Build history of the part. All positions in model axes, mm. Give positions to 0.01 mm unless a question says otherwise; leave off trailing zeros. Order: outer loops, then holes, each group sorted by start corner. A loop starts at its lowest first (then second) coordinate and runs counter-clockwise, first axis right, second up. Notation, with made-up numbers: (-34, 51.5) - (-26, 51.5) arc R25 ccw to (-26, 66.5) - close; hole circle Ø7 at (60, -30.75). An arc over 180 degrees is marked (long way). Answer in a Markdown table with one row per item.
```python
from build123d import *

# Parameters (mm, degrees)
BOSS_EXTRU_1_DEPTH      = 8
ENL_V_MAT_EXTRU_1_DEPTH = 4
CONG_2_R                = 10


with BuildPart() as part:
    # Esquisse1 → Boss.-Extru.1 (new body)
    with BuildSketch(Plane.XY):
        with BuildLine():
            Line((3.721082869, 15), (1.264283788, 21.75))
            Line((1.264283788, 21.75), (-1.264283788, 21.75))
            Line((-1.264283788, 21.75), (-3.721082869, 15))
            Line((-3.721082869, 15), (-53.721082869, 15))
            Line((-53.721082869, 15), (-53.721082869, -15))
            Line((-53.721082869, -15), (27.823144925, -15))
            Line((27.823144925, -15), (33.823144925, -19.5))
            ThreePointArc((33.823144925, -19.5), (35.323144925, -20), (36.823144925, -19.5))
            Line((36.823144925, -19.5), (42.823144925, -15))
            Line((42.823144925, -15), (148.823144925, -15))
            ThreePointArc((148.823144925, -15), (163.823144925, 0), (148.823144925, 15))
            Line((148.823144925, 15), (107.393640429, 15))
            Line((107.393640429, 15), (104.936841348, 21.75))
            Line((104.936841348, 21.75), (102.408273772, 21.75))
            Line((102.408273772, 21.75), (99.951474691, 15))
            Line((99.951474691, 15), (97.968862469, 15))
            Line((97.968862469, 15), (95.512063388, 21.75))
            Line((95.512063388, 21.75), (92.983495812, 21.75))
            Line((92.983495812, 21.75), (90.526696731, 15))
            Line((90.526696731, 15), (88.544084509, 15))
            Line((88.544084509, 15), (86.087285428, 21.75))
            Line((86.087285428, 21.75), (83.558717852, 21.75))
            Line((83.558717852, 21.75), (81.101918771, 15))
            Line((81.101918771, 15), (79.119306549, 15))
            Line((79.119306549, 15), (76.662507468, 21.75))
            Line((76.662507468, 21.75), (74.133939892, 21.75))
            Line((74.133939892, 21.75), (71.677140811, 15))
            Line((71.677140811, 15), (69.694528589, 15))
            Line((69.694528589, 15), (67.237729508, 21.75))
            Line((67.237729508, 21.75), (64.709161932, 21.75))
            Line((64.709161932, 21.75), (62.252362851, 15))
            Line((62.252362851, 15), (60.269750629, 15))
            Line((60.269750629, 15), (57.812951548, 21.75))
            Line((57.812951548, 21.75), (55.284383972, 21.75))
            Line((55.284383972, 21.75), (52.827584891, 15))
            Line((52.827584891, 15), (50.844972669, 15))
            Line((50.844972669, 15), (48.388173588, 21.75))
            Line((48.388173588, 21.75), (45.859606012, 21.75))
            Line((45.859606012, 21.75), (43.402806931, 15))
            Line((43.402806931, 15), (41.420194709, 15))
            Line((41.420194709, 15), (38.963395628, 21.75))
            Line((38.963395628, 21.75), (36.434828052, 21.75))
            Line((36.434828052, 21.75), (33.978028971, 15))
            Line((33.978028971, 15), (31.995416749, 15))
            Line((31.995416749, 15), (29.538617668, 21.75))
            Line((29.538617668, 21.75), (27.010050092, 21.75))
            Line((27.010050092, 21.75), (24.553251011, 15))
            Line((24.553251011, 15), (22.570638789, 15))
            Line((22.570638789, 15), (20.113839708, 21.75))
            Line((20.113839708, 21.75), (17.585272132, 21.75))
            Line((17.585272132, 21.75), (15.128473051, 15))
            Line((15.128473051, 15), (13.145860829, 15))
            Line((13.145860829, 15), (10.689061748, 21.75))
            Line((10.689061748, 21.75), (8.160494172, 21.75))
            Line((8.160494172, 21.75), (5.703695091, 15))
            Line((5.703695091, 15), (3.721082869, 15))
        make_face()
        with BuildLine():
            Line((-43.721082869, 3), (148.823144925, 3))
            ThreePointArc((148.823144925, 3), (151.823144925, 0), (148.823144925, -3))
            Line((148.823144925, -3), (-43.721082869, -3))
            ThreePointArc((-43.721082869, -3), (-46.721082869, 0), (-43.721082869, 3))
        make_face(mode=Mode.SUBTRACT)
    extrude(amount=BOSS_EXTRU_1_DEPTH)

    # Esquisse2 → Enlèv. mat.-Extru.1 (cut)
    with BuildSketch(Plane.XY.offset(8)):
        with BuildLine():
            Line((-43.721082869, 6), (148.823144925, 6))
            ThreePointArc((148.823144925, 6), (154.823144925, 0), (148.823144925, -6))
            Line((148.823144925, -6), (-43.721082869, -6))
            ThreePointArc((-43.721082869, -6), (-49.721082869, 0), (-43.721082869, 6))
        make_face()
    extrude(amount=-ENL_V_MAT_EXTRU_1_DEPTH, mode=Mode.SUBTRACT)

    # Congé2
    cong_2_edges = [part.edges().sort_by_distance(p)[0] for p in [
        (-53.721082869, -15, 4),
        (-53.721082869, 15, 4),
    ]]
    fillet(cong_2_edges, radius=CONG_2_R)


solid = part.part
```
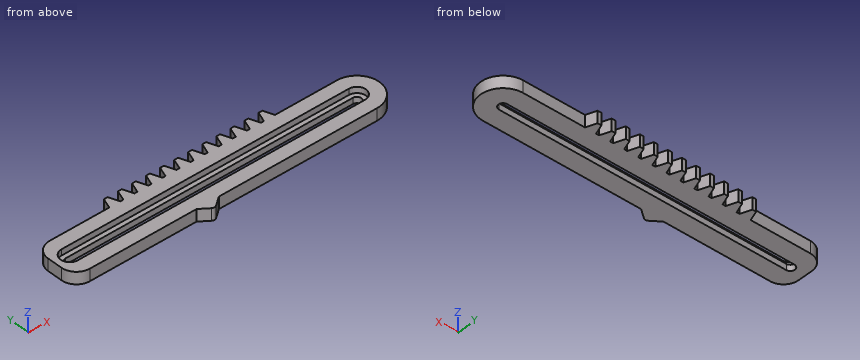
1. Cut at A-A on y = 0. Write the cut outline in (x, z), and give its area (3 significant figures).
Check result:
| item | result |
|---|---|
| outline | (-53.72, 0) - (-46.72, 0) - (-46.72, 4) - (-49.72, 4) - (-49.72, 8) - (-53.72, 8) - close; (151.82, 0) - (163.82, 0) - (163.82, 8) - (154.82, 8) - (154.82, 4) - (151.82, 4) - close |
| area | 128 mm² |
2. Drop flat-ended pins along their axis: P1, Ø5, axis at x = 8.5, y = 4.5, coming from the +Z side; P2, Ø0.6, axis at x = 80, z = 3, coming from the +Y side; P3, Ø1, axis at y = 9, z = 2.5, coming from the +X side; P4, Ø1, axis at x = 116.5, z = 5, coming from the -Y side. Give the stop position or say it passes through.
Check result:
| item | result |
|---|---|
| P1 | stops at z = 8 |
| P2 | stops at y = 15 |
| P3 | stops at x = 161.18 |
| P4 | stops at y = -15 |
3. Cut at C-C on y = -10.5. Write the cut outline in (x, z).
Check result:
| item | result |
|---|---|
| outline | (-52.07, 0) - (159.54, 0) - (159.54, 8) - (-52.07, 8) - close |
4. Probe line 1 (Y direction, x = 114, z = 7.5); line 2 (Y direction, x = 18, z = 5.75); line 3 (X direction, y = -5, z = 5.25). List the from-to ranges inside material, lowest first.
Check result:
| item | result |
|---|---|
| line 1 | y = -15 to -6, 6 to 15 |
| line 2 | y = -15 to -6, 6 to 21.75 |
| line 3 | x = -53.72 to -47.04, 152.14 to 162.97 |
5. Cut at B-B on x = -39.5. Write the cut outline in (y, z).
Check result:
| item | result |
|---|---|
| outline | (-15, 0) - (-3, 0) - (-3, 4) - (-6, 4) - (-6, 8) - (-15, 8) - close; (3, 0) - (15, 0) - (15, 8) - (6, 8) - (6, 4) - (3, 4) - close |
